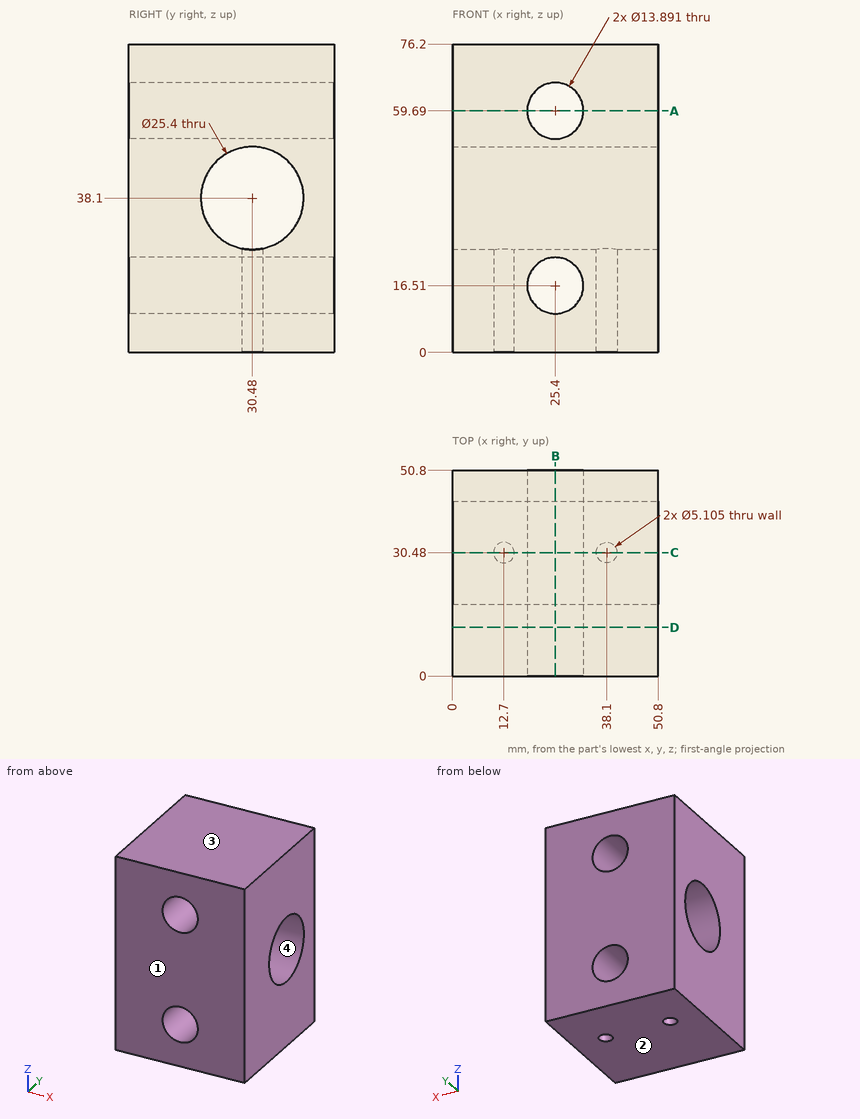
Here's the drawing with two shaded views (mm, measured from the low corner). I have some questions. Coordinates: 2 decimals unless noted, no trailing zeros. Order: outer loops, then holes, each group sorted by start corner. A loop starts at its lowest first (then second) coordinate and runs counter-clockwise, first axis right, second up.
Item 1: If we section it at A-A on z = 59.69: List the corners of the cut face in (x, y) for me (1 decimal).
Result sheet:
outline: (0, 0) - (18.5, 0) - (18.5, 50.8) - (0, 50.8) - close; (32.3, 0) - (50.8, 0) - (50.8, 50.8) - (32.3, 50.8) - close
Item 2: If we section it at D-D on y = 12: List the corners of the cut face in (x, z) for me (1 decimal), plus the area to 3 significant figures.
Result sheet:
outline: (0, 0) - (50.8, 0) - (50.8, 76.2) - (0, 76.2) - close; hole circle Ø13.9 at (25.4, 16.5); hole circle Ø13.9 at (25.4, 59.7)
area: 3,570 mm2
Item 3: I need wall thicknesses on line 1 (X direction, y = 12, z = 16); line 2 (Z direction, x = 41, y = 30.5); line 3 (Y direction, x = 38.5, z = 38.1). Which ranges of each line are inside material? Lowest first, please.
Result sheet:
line 1: x = 0 to 18.47, 32.33 to 50.8
line 2: z = 0 to 25.4, 50.8 to 76.2
line 3: y = 0 to 17.78, 43.18 to 50.8
Item 4: If we mould it in two halves opening along Z, with no side actions, what happens to the marked faces 1, 2, 3 and 4? For each: +Z half, -Z half, draft (parallel to the pull), parting line (faces both ways), or undercut.
Result sheet:
face 1: draft
face 2: -Z half
face 3: +Z half
face 4: undercut
Item 5: For P1, Ø3, axis at x = 12.7, y = 30.48, coming from the -Z side, with a flat end and sliding along its axis, tell me the tip position at first contact or that it passes through.
Result sheet:
P1: stops at z = 50.71
Item 6: If we section it at C-C on y = 30.48: List the corners of the cut face in (x, z) for me (1 decimal), plus the area to 3 significant figures.
Result sheet:
outline: (0, 0) - (10.1, 0) - (10.1, 25.4) - (0, 25.4) - close; (0, 50.8) - (50.8, 50.8) - (50.8, 76.2) - (0, 76.2) - close; (15.3, 0) - (35.5, 0) - (35.5, 25.4) - (15.3, 25.4) - close; (40.7, 0) - (50.8, 0) - (50.8, 25.4) - (40.7, 25.4) - close; hole circle Ø13.9 at (25.4, 16.5); hole circle Ø13.9 at (25.4, 59.7)
area: 2,020 mm2
Item 7: If we section it at B-B on x = 25.4: List the corners of the cut face in (y, z) for me (1 decimal), plus the area to 3 significant figures.
Result sheet:
outline: (0, 0) - (50.8, 0) - (50.8, 9.6) - (0, 9.6) - close; (0, 23.5) - (50.8, 23.5) - (50.8, 52.7) - (0, 52.7) - close; (0, 66.6) - (50.8, 66.6) - (50.8, 76.2) - (0, 76.2) - close; hole circle Ø25.4 at (30.5, 38.1)
area: 1,950 mm2
